Source: CAD feature listing. Evaluate the final solid. Frame: model axes, mm. A direction names the side the tool comes from. Round coordinates to 2 decimals unless told otherwise and drop trailing zeros. Loops run counter-clockwise (first coordinate to the right, second up) from the corner with the lowest first, then second, coordinate; pieces in that order, holes last. Notation, with made-up numbers: (59.25, -38.5) -> (98.25, -38.5) arc R25 ccw to (98.25, -6.5) -> close; hole circle Ø4 at (30.25, 42.5). An arc over 180 degrees is marked (long way). Write item = value, one per line.
from build123d import *

# Parameters (mm, degrees)
SKETCH1_W           = 200
SKETCH1_H           = 450
BOSS_EXTRUDE1_DEPTH = 16
SKETCH2_W           = 30
SKETCH2_H           = 30
CUT_EXTRUDE8_DEPTH  = 462.254810273
LPATTERN1_COUNT     = 7
LPATTERN1_PITCH     = 60
FILLET1_R           = 4


with BuildPart() as part:
    # Sketch1 → Boss-Extrude1 (new body)
    with BuildSketch(Plane.XY):
        with Locations((0, 225)):
            Rectangle(SKETCH1_W, SKETCH1_H)
    extrude(amount=BOSS_EXTRUDE1_DEPTH)

    # Sketch2 → Cut-Extrude8 (cut, symmetric)
    with BuildSketch(Plane.XY.offset(16)):
        with Locations((85, 40)):
            Rectangle(SKETCH2_W, SKETCH2_H)
    cut_extrude8 = extrude(amount=CUT_EXTRUDE8_DEPTH, both=True, mode=Mode.SUBTRACT)

    # LPattern1: Cut-Extrude8 ×7
    with Locations(*[(0, i * LPATTERN1_PITCH, 0) for i in range(1, LPATTERN1_COUNT)]):
        add(cut_extrude8, mode=Mode.SUBTRACT)

    # Fillet1
    fillet1_edges = [part.edges().sort_by_distance(p)[0] for p in [
        (70, 355, 8),
        (100, 355, 8),
        (100, 325, 8),
        (70, 325, 8),
        (70, 415, 8),
        (100, 415, 8),
        (100, 385, 8),
        (70, 385, 8),
        (70, 55, 8),
        (100, 55, 8),
        (100, 25, 8),
        (70, 25, 8),
        (70, 115, 8),
        (100, 115, 8),
        (100, 85, 8),
        (70, 85, 8),
        (70, 175, 8),
        (100, 175, 8),
        (100, 145, 8),
        (70, 145, 8),
        (-100, 450, 8),
        (100, 450, 8),
        (100, 0, 8),
        (-100, 0, 8),
        (70, 235, 8),
        (100, 235, 8),
        (100, 205, 8),
        (70, 205, 8),
        (70, 295, 8),
        (100, 295, 8),
        (100, 265, 8),
        (70, 265, 8),
    ]]
    fillet(fillet1_edges, radius=FILLET1_R)


solid = part.part
1. Mould query, pull axis Y, two halves, no side actions, for faces 1 (the face through (100, 432, 8)), 2 (the face through (-1, 0, 8)), 3 (the face through (70, 400, 8)), 4 (the face through (85, 385, 8)). Classes: released by +Y, released by -Y, zero draft, split by the parting line, or undercut.
Evaluation:
face_1 = zero draft
face_2 = released by -Y
face_3 = undercut
face_4 = undercut
2. Contact query for a flat-ended pin moving along its axis: pin 1 Ø8 at (y, z) = (281.5, 6.5) entering from +X. Output: stop coordinate, or through.
Evaluation:
pin_1 = 70
3. Set-up query: faces 5 (the face through (100, 70, 8)), 6 (the face through (85, 295, 8)). Return all of +Z, -Z, +X, -X, +Y, -Y with unobstructed straight access to the full face (end or side cutting, diameter ignored); none if empty.
Evaluation:
face_5 = +Z, -Z, +X, +Y, -Y
face_6 = +Z, -Z, +X
4. Section query A-A (x = 85.5). Give the number of separate pieces and of enclosed holes in the cut face, then the cut area to 3 significant figures.
Evaluation:
separate_pieces = 8
enclosed_holes = 0
area = 3,840 mm²
5. Section query B-B (y = 283.5). Return the cut outline in (x, z).
Evaluation:
outline = (-100, 0) -> (70, 0) -> (70, 16) -> (-100, 16) -> close
6. Line query: probe 1 along X at (y, z) = (344, 1.75); probe 2 along X at (y, z) = (263.5, 15.25). Output: solid intervals per line, ascending. Write a range as from..to.
Evaluation:
probe_1 = -100..70
probe_2 = -100..99.12
